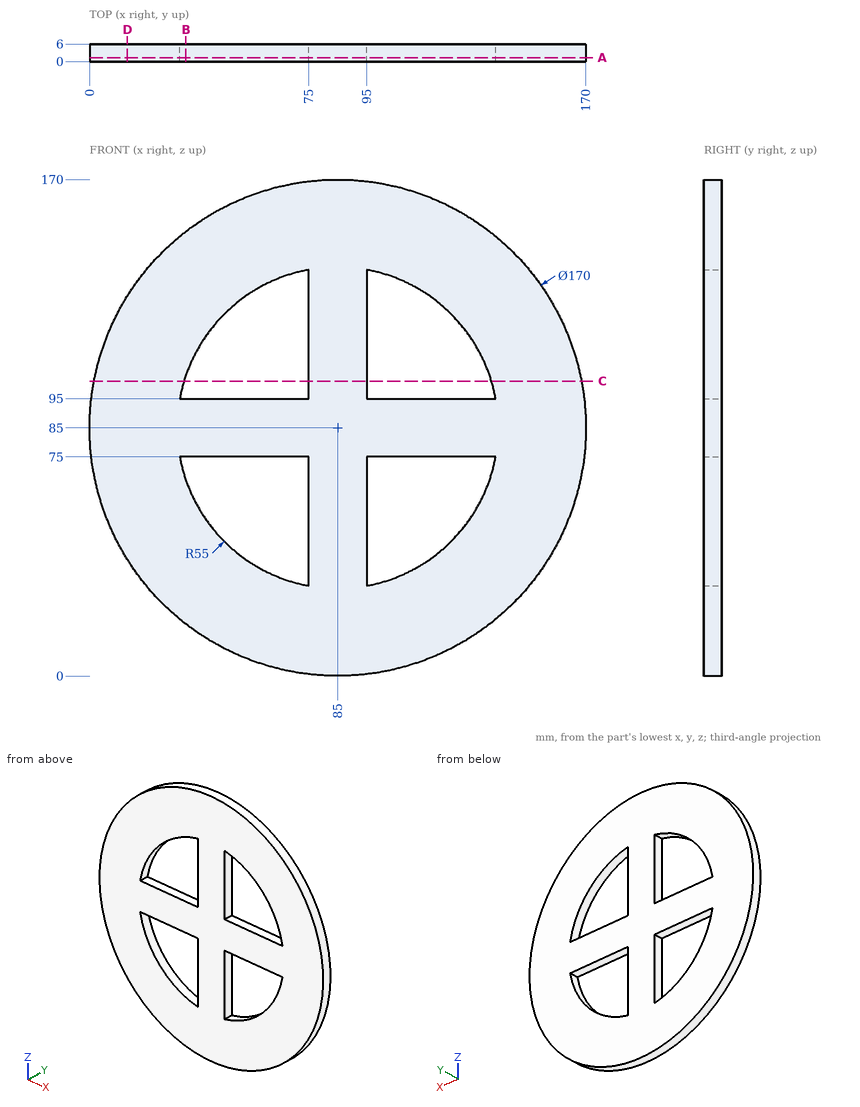
Design review of the part shown in the three views and the two pictorial views. Dimensions are in mm from the part's minimum x, y and z. Give positions to 0.01 mm unless a question says otherwise; leave off trailing zeros. Loops run counter-clockwise (first coordinate to the right, second up) from the corner with the lowest first, then second, coordinate; pieces in that order, holes last. Notation, with made-up numbers: (31.25, -30.5) -> (86.25, -30.5) arc R22 cw to (86.25, -8.5) -> close; hole circle Ø10 at (5.25, -33). An arc over 180 degrees is marked (long way). One line per item, written item: value.
Q1. We need section A-A on y = 1.3. Give the boundary of the cut face in (x, z).
Numbers:
outline: circle Ø170 at (85, 85); hole (30.92, 75) arc R55 ccw to (75, 30.92) -> (75, 75) -> close; hole (30.92, 95) -> (75, 95) -> (75, 139.08) arc R55 ccw to start; hole (95, 30.92) arc R55 ccw to (139.08, 75) -> (95, 75) -> close; hole (95, 95) -> (139.08, 95) arc R55 ccw to (95, 139.08) -> close
Q2. For L1, parallel to X at y = 3.1, z = 106; L2, parallel to X at y = 0.35, z = 99.5; L3, parallel to Z at x = 64.5, y = 0.75, list the stretches that pass through material, from the lowest coordinate up.
Numbers:
L1: x = 2.63 to 34.17, 75 to 95, 135.83 to 167.37
L2: x = 1.25 to 31.95, 75 to 95, 138.05 to 168.75
L3: z = 2.51 to 33.96, 75 to 95, 136.04 to 167.49
Q3. We need section B-B on x = 33. Give the boundary of the cut face in (y, z), and give its area (3 significant figures).
Numbers:
outline: (0, 17.76) -> (6, 17.76) -> (6, 67.08) -> (0, 67.08) -> close; (0, 75) -> (6, 75) -> (6, 95) -> (0, 95) -> close; (0, 102.92) -> (6, 102.92) -> (6, 152.24) -> (0, 152.24) -> close
area: 712 mm^2
Q4. We need section C-C on z = 101. Give the boundary of the cut face in (x, y), and give its area (3 significant figures).
Numbers:
outline: (1.52, 0) -> (32.38, 0) -> (32.38, 6) -> (1.52, 6) -> close; (75, 0) -> (95, 0) -> (95, 6) -> (75, 6) -> close; (137.62, 0) -> (168.48, 0) -> (168.48, 6) -> (137.62, 6) -> close
area: 490 mm^2
Q5. For pin 1 Ø1.8 at (x, y) = (49, 3) entering from +Z; pin 2 Ø2 at (x, y) = (59.5, 3.5) entering from +Z; pin 3 Ø3 at (y, z) = (3, 47) entering from +X, all flat-tipped, find the tip position at first contact; note any pin that passes through.
Numbers:
pin 1: stops at z = 162.41
pin 2: stops at z = 166.39
pin 3: stops at x = 161.76
Q6. We need section D-D on x = 13. Give the boundary of the cut face in (y, z).
Numbers:
outline: (0, 39.82) -> (6, 39.82) -> (6, 130.18) -> (0, 130.18) -> close
